Here's how the part is built. I have some questions about the finished solid (model axes, mm). Give positions to 0.01 mm unless a question says otherwise; leave off trailing zeros. Write each loop counter-clockwise with the first axis right and the second up, starting at its lowest first coordinate (ties: lowest second). Pieces come first, ordered by that corner, then holes. Notation, with made-up numbers: (41.25, 32) -> (74.25, 32) arc R15 cw to (74.25, 38) -> close; hole circle Ø1 at (47, 29). An arc over 180 degrees is marked (long way). Return JSON: item names as keys, results as strings.
from build123d import *

# Parameters (mm, degrees)
F0_W     = 130
F0_H     = 130
F1_DEPTH = 25


with BuildPart() as f1:
    # F0 (on Top) → F1 (new body)
    with BuildSketch(Plane.XY):
        with Locations((-0.584693, 3.311556)):
            Rectangle(F0_W, F0_H)
        with BuildLine():
            Line((-15.594432, 54.811556), (-9.594432, 54.811556))
            Line((-9.594432, 54.811556), (-9.594432, 52.311556))
            Line((-9.594432, 52.311556), (-12.594432, 52.311556))
            Line((-12.594432, 52.311556), (-42.41335, -45.22173))
            Line((-42.41335, -45.22173), (-37.91335, -45.22173))
            Line((-37.91335, -45.22173), (-29.92532, -19.09406))
            Line((-29.92532, -19.09406), (-21.92532, -19.09406))
            Line((-21.92532, -19.09406), (-21.92532, -45.09406))
            Line((-21.92532, -45.09406), (-17.42532, -45.09406))
            Line((-17.42532, -45.09406), (-17.42532, 29.40594))
            Line((-17.42532, 29.40594), (1.170036, 29.40594))
            ThreePointArc((1.170036, 29.40594), (11.137538, 25.758417), (16.396462, 16.538914))
            Line((16.396462, 16.538914), (16.663941, -29.106018))
            ThreePointArc((16.663941, -29.106018), (11.736324, -39.489004), (1.045823, -43.708128))
            Line((1.045823, -43.708128), (-6.094494, -43.708128))
            Line((-6.094494, -43.708128), (-6.094494, -44.908128))
            Line((-6.094494, -44.908128), (20.69909, -44.908128))
            Line((20.69909, -44.908128), (20.69909, -18.908128))
            Line((20.69909, -18.908128), (28.69909, -18.908128))
            Line((28.69909, -18.908128), (36.84589, -45.55511))
            Line((36.84589, -45.55511), (41.34589, -45.55511))
            Line((41.34589, -45.55511), (11.425047, 52.311556))
            Line((11.425047, 52.311556), (8.425047, 52.311556))
            Line((8.425047, 52.311556), (8.425047, 54.811556))
            Line((8.425047, 54.811556), (14.425047, 54.811556))
            Line((14.425047, 54.811556), (45.915307, -48.188444))
            Line((45.915307, -48.188444), (33.915307, -48.188444))
            Line((33.915307, -48.188444), (25.660579, -21.188444))
            Line((25.660579, -21.188444), (23.660579, -21.188444))
            Line((23.660579, -21.188444), (23.660579, -48.188444))
            Line((23.660579, -48.188444), (-9.339421, -48.188444))
            Line((-9.339421, -48.188444), (-9.339421, -39.988444))
            Line((-9.339421, -39.988444), (1.045823, -39.988444))
            ThreePointArc((1.045823, -39.988444), (9.070223, -36.852271), (12.841448, -29.106018))
            Line((12.841448, -29.106018), (13.222281, 16.538914))
            ThreePointArc((13.222281, 16.538914), (8.928276, 23.561392), (1.170036, 26.311556))
            Line((1.170036, 26.311556), (-13.829964, 26.311556))
            Line((-13.829964, 26.311556), (-13.829964, -48.188444))
            Line((-13.829964, -48.188444), (-24.829964, -48.188444))
            Line((-24.829964, -48.188444), (-24.829964, -21.188444))
            Line((-24.829964, -21.188444), (-26.829964, -21.188444))
            Line((-26.829964, -21.188444), (-35.084693, -48.188444))
            Line((-35.084693, -48.188444), (-47.084693, -48.188444))
            Line((-47.084693, -48.188444), (-15.594432, 54.811556))
        make_face(mode=Mode.SUBTRACT)
    extrude(amount=F1_DEPTH)


solid = f1.part
1. If I drill on line 1 (X direction, y = -4, z = 21); line 2 (X direction, y = 0.5, z = 10.5); line 3 (Y direction, x = 2.5, z = 9.5), over which ranges is the centre line in solid material (lowest first)? Write a range as [from, to].
Taken from the geometry:
{"line 1": "x = [-65.58, -33.57], [-29.81, -17.43], [-13.83, 13.05], [16.52, 28.64], [32.41, 64.42]", "line 2": "x = [-65.58, -32.2], [-28.43, -17.43], [-13.83, 13.09], [16.49, 27.27], [31.03, 64.42]", "line 3": "y = [-61.69, -48.19], [-44.91, -43.64], [-39.9, 26.24], [29.35, 68.31]"}
2. If we mould it in two halves opening along X, with no side actions, what happens to faces 1 (the face through (64.415, 2, 12)), 2 (the face through (-27.295, 4.228, 12.325))? For each: released by +X, released by -X, zero draft, split by the parting line, or undercut.
Taken from the geometry:
{"face 1": "released by +X", "face 2": "undercut"}
3. Suppose I cut it at A-A, the plane y = 40.5. List the corners of the cut face in (x, z) for me, and give its area (3 significant figures).
Taken from the geometry:
{"outline": "(-65.58, 0) -> (-19.97, 0) -> (-19.97, 25) -> (-65.58, 25) -> close; (-16.21, 0) -> (15.04, 0) -> (15.04, 25) -> (-16.21, 25) -> close; (18.8, 0) -> (64.42, 0) -> (64.42, 25) -> (18.8, 25) -> close", "area": "3,060 mm²"}
4. Suppose I cut it at C-C, the plane y = -31. Count the separate pieces of the cut face and the enclosed holes in it, and give its area (3 significant figures).
Taken from the geometry:
{"separate pieces": "9", "enclosed holes": "0", "area": "2,540 mm²"}
5. Suppose I cut it at B-B, the plane y = -7. List the corners of the cut face in (x, z) for me, and give its area (3 significant figures).
Taken from the geometry:
{"outline": "(-65.58, 0) -> (-34.49, 0) -> (-34.49, 25) -> (-65.58, 25) -> close; (-30.73, 0) -> (-17.43, 0) -> (-17.43, 25) -> (-30.73, 25) -> close; (-13.83, 0) -> (13.03, 0) -> (13.03, 25) -> (-13.83, 25) -> close; (16.53, 0) -> (29.56, 0) -> (29.56, 25) -> (16.53, 25) -> close; (33.32, 0) -> (64.42, 0) -> (64.42, 25) -> (33.32, 25) -> close", "area": "2,880 mm²"}
